```python
from build123d import *

# Parameters (mm, degrees)
SKETCH2_R           = 609.6
BOSS_EXTRUDE2_DEPTH = 76.2
CUT_EXTRUDE1_DEPTH  = 77.2
CIRPATTERN1_COUNT   = 30


with BuildPart() as part:
    # Sketch2 → Boss-Extrude2 (new body)
    with BuildSketch(Plane.XY):
        Circle(SKETCH2_R)
    extrude(amount=BOSS_EXTRUDE2_DEPTH)

    # Sketch3 → Cut-Extrude1 (cut, through all)
    with BuildSketch(Plane.XY.offset(76.2)):
        with BuildLine():
            ThreePointArc((24.912616177, 523.282311167), (0, 523.875), (-24.912616177, 523.282311167))
            ThreePointArc((-24.912616177, 523.282311167), (-35.087110683, 567.908462249), (-59.380088455, 606.701050844))
            ThreePointArc((-59.380088455, 606.701050844), (0, 609.6), (59.380088455, 606.701050844))
            ThreePointArc((59.380088455, 606.701050844), (37.988368572, 566.709702519), (24.912616177, 523.282311167))
        make_face()
    cut_extrude1 = extrude(amount=-CUT_EXTRUDE1_DEPTH, mode=Mode.SUBTRACT)

    # CirPattern1: Cut-Extrude1 ×30 about axis
    cirpattern1_axis = Axis((-0.006195071, -3.21023047, 0), (0, 0, 1))
    for i in range(1, CIRPATTERN1_COUNT):
        add(cut_extrude1.rotate(cirpattern1_axis, i * 360 / CIRPATTERN1_COUNT), mode=Mode.SUBTRACT)


solid = part.part
```
Source: CAD feature listing. Evaluate the final solid. Frame: model axes, mm. A direction names the side the tool comes from. Coordinates: 2 decimals unless noted, no trailing zeros. Order: outer loops, then holes, each group sorted by start corner. A loop starts at its lowest first (then second) coordinate and runs counter-clockwise, first axis right, second up. Notation, with made-up numbers: M 71,5 L 126,5 A31 ccw 126,42 Z; hole C 47.25,-37.75 d10. An arc over 180 degrees is marked long. Write each question's results on one line, items separated by ' | '. Start each with the question number.
1) Line query: line 1 (X direction, y = 539, z = 46); line 2 (X direction, y = 474.5, z = 66); line 3 (Y direction, x = -466.5, z = 9). Output: solid intervals per line, ascending. Write a range as from..to.
2) Contact query for flat-ended pins moving along their axis: pin 1 Ø1.5 at (x, z) = (-265, 39.5) entering from +Y; pin 2 Ø4 at (y, z) = (-148.5, 48) entering from -X; pin 3 Ø10 at (x, z) = (168.5, 54.5) entering from +Y. Output: stop coordinate, or through.
3) Draft query along X for faces 5 (the face through (-529.93, 208.73, 38.63)), 6 (the face through (365.88, 435.63, 38.63)), 7 (the face through (476.165, 311.582, 38.633)). Return one class per face: released by +X, released by -X, zero draft, split by the parting line, or undercut.
4) Section query B-B (y = 214). Return the cut outline in (x, z), plus the area to 3 significant figures.
5) Section query A-A (x = -251.5). Return the cut outline in (y, z).
6) Access query for faces 1 (the face through (38.232, 567.297, 38.633)), 2 (the face through (261.307, -507.714, 38.633)), 3 (the face through (-524.167, 52.238, 38.633)), 4 (the face through (-85.173, -564.733, 38.633)). Directions: +Z, -Z, +X, -X, +Y, -Y. A direction counts if a zero-diameter tool reaches every point of the face in a straight line with its end or side. Return the directions, or none.
Answers:
1) line 1: x = -197.19..-147.31, -84.39..-26.72, 28.57..86.69, 150.81..200.27 | line 2: x = -302.81..-240.69, -222.74..222.73, 241.92..306.02 | line 3: y = -361.77..-306.96, -248.57..242.15, 304.74..358.04
2) pin 1: stops at y = 505.58 | pin 2: stops at x = -507.24 | pin 3: stops at y = 569.14
3) face 5: released by -X | face 6: undercut | face 7: released by +X
4) outline: M -535.92,0 L 540.29,0 L 540.29,76.2 L -535.92,76.2 Z | area: 82,000 mm^2
5) outline: M -492.7,0 L 490.23,0 L 490.23,76.2 L -492.7,76.2 Z
6) face 1: +Z, -Z, +Y | face 2: +Z, -Z, -Y | face 3: +Z, -Z, -X | face 4: +Z, -Z
